Read the model definition and answer for the solid it produces. Units are mm, in the model's axes. Face numbers are marked on the shaded views. Give positions to 0.01 mm unless a question says otherwise; leave off trailing zeros. Order: outer loops, then holes, each group sorted by start corner. A loop starts at its lowest first (then second) coordinate and runs counter-clockwise, first axis right, second up. Notation, with made-up numbers: (11.5, 35.25) - (69.5, 35.25) arc R9 ccw to (69.5, 47.25) - close; hole circle Ø7 at (-23, -22). An arc over 180 degrees is marked (long way). Write item = value, one per line.
```python
from build123d import *

# Parameters (mm, degrees)
SKETCH_1_W        = 10
SKETCH_1_H        = 2.5
HOLE_WIZARD_M31_D = 2.5
CHAMFER_1_SIZE    = 0.2
CHAMFER_2_SIZE    = 0.5


with BuildPart() as part:
    # Эскиз1 → Повернуть1 (revolve)
    with BuildSketch(Plane.XY):
        with Locations((5, 1.25)):
            Rectangle(SKETCH_1_W, SKETCH_1_H)
    revolve(axis=Axis((10, 0, 0), (-1, 0, 0)))

    # Отверстие обработанное метчиком M31 (through all)
    with Locations(Plane(origin=(10, 0, 0), x_dir=(0, 0, -1), z_dir=(1, 0, 0))):
        with Locations((0, 0)):
            Hole(HOLE_WIZARD_M31_D / 2)

    # Фаска1
    chamfer_1_edges = [part.edges().sort_by_distance(p)[0] for p in [
        (10, 0, -1.25),
        (0, 0, -1.25),
    ]]
    chamfer(chamfer_1_edges, length=CHAMFER_1_SIZE)

    # Фаска2
    chamfer_2_edges = [part.edges().sort_by_distance(p)[0] for p in [
        (10, -2.5, 0),
        (0, -2.5, 0),
    ]]
    chamfer(chamfer_2_edges, length=CHAMFER_2_SIZE)


solid = part.part
```
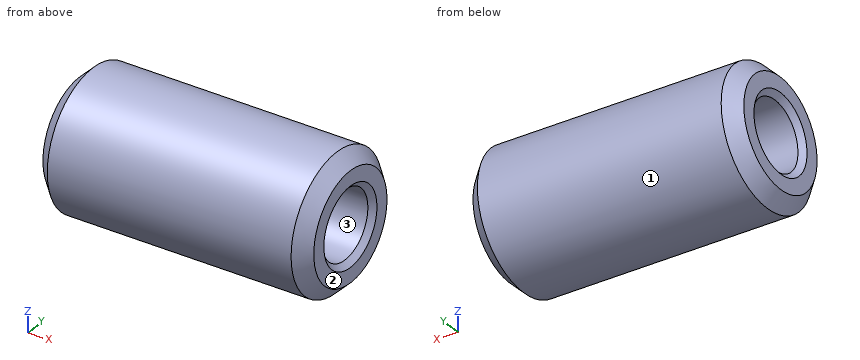
1. Straight lines are drawn through the part: L1, parallel to Y at x = 5, z = 0; L2, parallel to Z at x = 2, y = -0.5; L3, parallel to Z at x = 6.25, y = -0.15. For each, find the intervals that lie inside material, in ascending order. Write a range as [from, to].
Recorded:
L1 = [-2.5, -1.25], [1.25, 2.5]
L2 = [-2.45, -1.15], [1.15, 2.45]
L3 = [-2.5, -1.24], [1.24, 2.5]
2. A flat-ended cylindrical pin translates along its axis: pin 1 (3 mm diameter, centred on x = 8, z = -2, fed in from -Y). Find the tip coordinate at first contact, or state that the pin passes through.
Recorded:
pin_1 = -2.45
3. Section C-C (x = 4.75) is taken. Determine the outline of the cut face in (y, z).
Recorded:
outline = circle Ø5 at (0, 0); hole circle Ø2.5 at (0, 0)
4. Determine the mould class of the marked faces 1, 2 and 3 for opening direction Z: +Z half, -Z half, draft (parallel to the pull), parting line (faces both ways), or undercut.
Recorded:
face_1 = parting line
face_2 = draft
face_3 = undercut
5. Section A-A (z = 0) is taken. Determine the outline of the cut face in (x, y), and give its area (3 significant figures).
Recorded:
outline = (0, -2) - (0.5, -2.5) - (9.5, -2.5) - (10, -2) - (10, -1.45) - (9.8, -1.25) - (0.2, -1.25) - (0, -1.45) - close; (0, 1.45) - (0.2, 1.25) - (9.8, 1.25) - (10, 1.45) - (10, 2) - (9.5, 2.5) - (0.5, 2.5) - (0, 2) - close
area = 24.4 mm^2
